Part print with two shaded views. Sizes in mm from the minimum x, y, z corner. A direction names the side the tool comes from. Give positions to 0.01 mm unless a question says otherwise; leave off trailing zeros. Write each loop counter-clockwise with the first axis right and the second up, starting at its lowest first coordinate (ties: lowest second). Pieces come first, ordered by that corner, then holes. Notation, with made-up numbers: (84, 74) - (119, 74) arc R10 ccw to (119, 91) - close; hole circle Ø7 at (-35, 33). An arc over 180 degrees is marked (long way). One line per item, written item: value. Start each with the question number.
(1) Cut at C-C, the plane x = 29. List the corners of the cut face in (y, z) (1 decimal), and give its area (3 significant figures).
(2) Probe L1, parallel to Y at x = 11.5, z = 5; L2, parallel to X at y = 11.75, z = 1.5; L3, parallel to X at y = 7.75, z = 7 (1 decimal). List the from-to ranges inside material, lowest first.
(3) Cut at B-B, the plane y = 15.5. List the corners of the cut face in (x, z), and give its area (3 significant figures).
(4) Cut at D-D, the plane y = 7.5. List the corners of the cut face in (x, z) (1 decimal).
(5) 3-axis set-ups, long thin cutter, end or side, ignore diameter. For the marked faces 1, 2, 3 and 4: which of +Z, -Z, +X, -X, +Y, -Y reach the whole face in a straight line?
(6) Drop flat-ended pins along their axis: P1, Ø2, axis at y = 7.5, z = 6, coming from the -X side; P2, Ø1, axis at y = 7.5, z = 6, coming from the -X side; P3, Ø1.5, axis at x = 60.5, z = 7.5, coming from the -Y side. Give the stop position or say it passes through.
(7) Cut at A-A, the plane z = 9.25. List the corners of the cut face in (x, y), and give its area (3 significant figures).
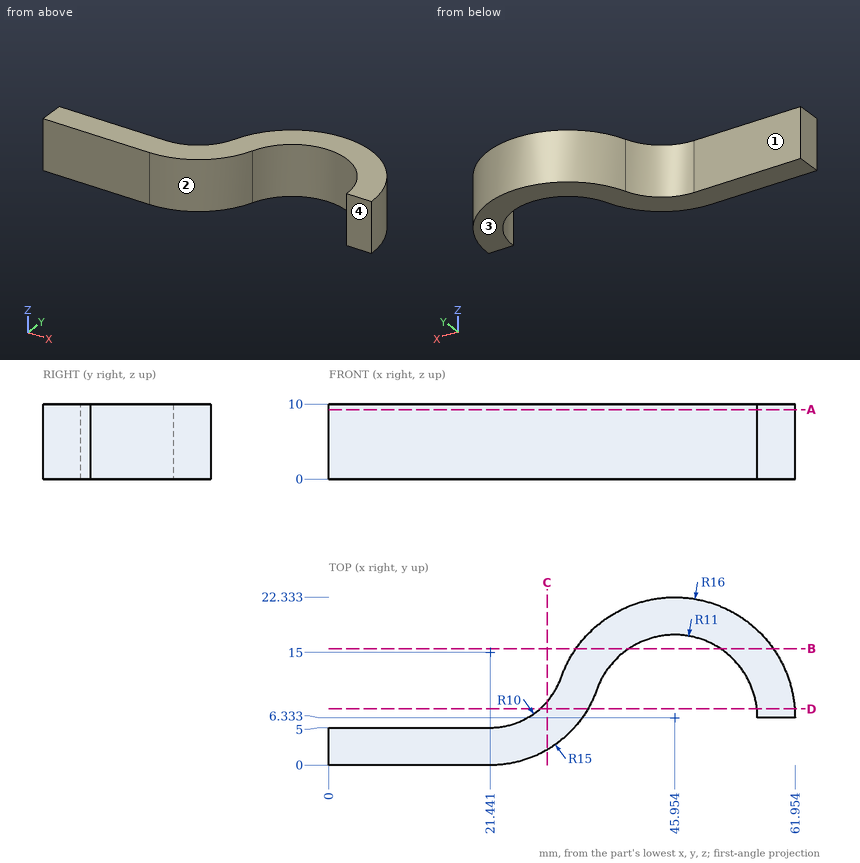
Answers follow:
1. outline: (2, 0) - (8.5, 0) - (8.5, 10) - (2, 10) - close
1. area: 64.1 mm²
2. L1: y = 0 to 5
2. L2: x = 30.9 to 36.38, 55.53 to 61.01
2. L3: x = 28.3 to 34.6, 56.9 to 61.9
3. outline: (32.84, 0) - (39.87, 0) - (39.87, 10) - (32.84, 10) - close; (52.03, 0) - (59.07, 0) - (59.07, 10) - (52.03, 10) - close
3. area: 141 mm²
4. outline: (28.1, 0) - (34.4, 0) - (34.4, 10) - (28.1, 10) - close; (56.9, 0) - (61.9, 0) - (61.9, 10) - (56.9, 10) - close
5. face 1: +Z, -Z, -X, +Y
5. face 2: +Z, -Z, -Y
5. face 3: -Z, +X, -X, +Y, -Y
5. face 4: +Z, -Z, +X, -Y
6. P1: stops at x = 26.71
6. P2: stops at x = 27.44
6. P3: stops at y = 6.33
7. outline: (0, 0) - (21.44, 0) arc R15 ccw to (35.58, 10) arc R11 cw to (56.95, 6.33) - (61.95, 6.33) arc R16 ccw to (30.87, 11.67) arc R10 cw to (21.44, 5) - (0, 5) - close
7. area: 373 mm²
